Could you check a few things on this model? Use its own coordinates, in mm. A direction names the side the tool comes from. Round coordinates to 2 decimals unless told otherwise and drop trailing zeros. Loops run counter-clockwise (first coordinate to the right, second up) from the corner with the lowest first, then second, coordinate; pieces in that order, holes last. Notation, with made-up numbers: (51.25, 38) -> (92.25, 38) arc R25 ccw to (92.25, 74) -> close; hole circle Ø6 at (41.5, 17.25). An arc over 180 degrees is marked (long way). Put each result on its own line as item: value. Start each with the question number.
1. I need wall thicknesses on line 1 (Y direction, x = 134, z = 2.2); line 2 (Y direction, x = 156, z = 0.7); line 3 (Y direction, x = 65, z = 2.1). Which ranges of each line are inside material? Lowest first, please. Write a range as [from, to].
2. Imagine slicing it at C-C, the plane z = 1.3. Count the separate pieces of the cut face and the enclosed holes in it, and give its area (3 significant figures).
3. Imagine slicing it at D-D, the plane x = 124. Please give me the cut outline in (y, z) (3 decimals), and give its area (3 significant figures).
4. Imagine slicing it at A-A, the plane x = 141.5. Please give me the cut outline in (y, z) (3 decimals), and give its area (3 significant figures).
5. Which directions (+Z, -Z, +X, -X, +Y, -Y) give clear straight access to the entire face, cutting with the end or side of a thin tool? Please do faces 4 (the cylindrical face through (165.083, -51.404, 1.565)), 5 (the flat face through (148.274, 233.48, 1.61)), 6 (the cylindrical face through (84.258, 200.735, 1.565)).
6. If we mould it in two halves opening along Y, with no side actions, what happens to faces 1 (the flat face through (102, 121, 3.175)), 2 (the cylindrical face through (40.237, 288.703, 1.565)), 3 (the flat face through (56.584, 233.942, 1.61))? For each: pulls with the +Y half, pulls with the -Y half, needs draft (parallel to the pull), parting line crosses it, or undercut.
7. Imagine slicing it at B-B, the plane y = 99. Please give me the cut outline in (x, z) (3 decimals).
8. I'm going to push flat-ended pins straight in: P1, Ø1.5, axis at y = 10, z = 1, coming from the -X side; P2, Ø1.6, axis at y = 146, z = 1.5, coming from the -X side; P3, Ø1, axis at y = 134, z = 2, coming from the +X side. Where does each tip first touch, or does it pass through?
```python
from build123d import *

# Parameters (mm, degrees)
BOSS_EXTRUDE1_DEPTH = 3.175
CUT_EXTRUDE1_DEPTH  = 10
SKETCH3_R           = 2.0193
BOSS_EXTRUDE2_DEPTH = 3.175
FILLET1_R           = 10
FILLET2_R           = 50
SKETCH4_R           = 2.02
CUT_EXTRUDE2_DEPTH  = 10


with BuildPart() as part:
    # Sketch1 → Boss-Extrude1 (new body)
    with BuildSketch(Plane.XY):
        Polygon((165.934536959, -16.66935), (157.315236959, -8.05005), (115.359952094, -8.05005), (89.959952094, -8.05005), (48.004667228, -8.05005), (39.385367228, -16.66935), (39.385367228, -40.05005), (39.385367228, -52.41105), (165.934536959, -56.67505), (165.934536959, -42.05005), align=None)
        with BuildLine():
            ThreePointArc((47.685367228, -44.38075), (49.704667228, -46.40005), (47.685367228, -48.41935))
            ThreePointArc((47.685367228, -48.41935), (45.666067228, -46.40005), (47.685367228, -44.38075))
        make_face(mode=Mode.SUBTRACT)
        with BuildLine():
            ThreePointArc((47.685367228, -12.63075), (49.704667228, -14.65005), (47.685367228, -16.66935))
            ThreePointArc((47.685367228, -16.66935), (45.666067228, -14.65005), (47.685367228, -12.63075))
        make_face(mode=Mode.SUBTRACT)
        with BuildLine():
            ThreePointArc((73.085367228, -44.38075), (75.104667228, -46.40005), (73.085367228, -48.41935))
            ThreePointArc((73.085367228, -48.41935), (71.066067228, -46.40005), (73.085367228, -44.38075))
        make_face(mode=Mode.SUBTRACT)
        with BuildLine():
            ThreePointArc((73.085367228, -12.63075), (75.104667228, -14.65005), (73.085367228, -16.66935))
            ThreePointArc((73.085367228, -16.66935), (71.066067228, -14.65005), (73.085367228, -12.63075))
        make_face(mode=Mode.SUBTRACT)
        with BuildLine():
            ThreePointArc((132.234536959, -44.38075), (134.253836959, -46.40005), (132.234536959, -48.41935))
            ThreePointArc((132.234536959, -48.41935), (130.215236959, -46.40005), (132.234536959, -44.38075))
        make_face(mode=Mode.SUBTRACT)
        with BuildLine():
            ThreePointArc((132.234536959, -12.63075), (134.253836959, -14.65005), (132.234536959, -16.66935))
            ThreePointArc((132.234536959, -16.66935), (130.215236959, -14.65005), (132.234536959, -12.63075))
        make_face(mode=Mode.SUBTRACT)
        with BuildLine():
            ThreePointArc((157.634536959, -44.38075), (159.653836959, -46.40005), (157.634536959, -48.41935))
            ThreePointArc((157.634536959, -48.41935), (155.615236959, -46.40005), (157.634536959, -44.38075))
        make_face(mode=Mode.SUBTRACT)
        with BuildLine():
            ThreePointArc((157.634536959, -12.63075), (159.653836959, -14.65005), (157.634536959, -16.66935))
            ThreePointArc((157.634536959, -16.66935), (155.615236959, -14.65005), (157.634536959, -12.63075))
        make_face(mode=Mode.SUBTRACT)
        Polygon((115.359952094, -8.05005), (157.315236959, -8.05005), (115.359952094, 33.905234866), align=None)
        Polygon((89.959952094, -8.05005), (115.359952094, -8.05005), (115.359952094, 33.905234866), (115.359952094, 203.394265134), (115.359952094, 245.34955), (89.959952094, 245.34955), (89.959952094, 203.394265134), (89.959952094, 33.905234866), align=None)
        Polygon((48.004667228, -8.05005), (89.959952094, -8.05005), (89.959952094, 33.905234866), align=None)
        Polygon((89.959952094, 245.34955), (115.359952094, 245.34955), (157.315236959, 245.34955), (165.934536959, 253.96885), (165.934536959, 279.34955), (165.934536959, 293.97455), (39.385367228, 289.71055), (39.385367228, 277.34955), (39.385367228, 253.96885), (48.004667228, 245.34955), align=None)
        with BuildLine():
            ThreePointArc((47.685367228, 253.96885), (49.704667228, 251.94955), (47.685367228, 249.93025))
            ThreePointArc((47.685367228, 249.93025), (45.666067228, 251.94955), (47.685367228, 253.96885))
        make_face(mode=Mode.SUBTRACT)
        with BuildLine():
            ThreePointArc((47.685367228, 285.71885), (49.704667228, 283.69955), (47.685367228, 281.68025))
            ThreePointArc((47.685367228, 281.68025), (45.666067228, 283.69955), (47.685367228, 285.71885))
        make_face(mode=Mode.SUBTRACT)
        with BuildLine():
            ThreePointArc((73.085367228, 253.96885), (75.104667228, 251.94955), (73.085367228, 249.93025))
            ThreePointArc((73.085367228, 249.93025), (71.066067228, 251.94955), (73.085367228, 253.96885))
        make_face(mode=Mode.SUBTRACT)
        with BuildLine():
            ThreePointArc((73.085367228, 285.71885), (75.104667228, 283.69955), (73.085367228, 281.68025))
            ThreePointArc((73.085367228, 281.68025), (71.066067228, 283.69955), (73.085367228, 285.71885))
        make_face(mode=Mode.SUBTRACT)
        with BuildLine():
            ThreePointArc((132.234536959, 253.96885), (134.253836959, 251.94955), (132.234536959, 249.93025))
            ThreePointArc((132.234536959, 249.93025), (130.215236959, 251.94955), (132.234536959, 253.96885))
        make_face(mode=Mode.SUBTRACT)
        with BuildLine():
            ThreePointArc((157.634536959, 253.96885), (159.653836959, 251.94955), (157.634536959, 249.93025))
            ThreePointArc((157.634536959, 249.93025), (155.615236959, 251.94955), (157.634536959, 253.96885))
        make_face(mode=Mode.SUBTRACT)
        with BuildLine():
            ThreePointArc((157.634536959, 285.71885), (159.653836959, 283.69955), (157.634536959, 281.68025))
            ThreePointArc((157.634536959, 281.68025), (155.615236959, 283.69955), (157.634536959, 285.71885))
        make_face(mode=Mode.SUBTRACT)
        Polygon((115.359952094, 245.34955), (115.359952094, 203.394265134), (157.315236959, 245.34955), align=None)
        Polygon((48.004667228, 245.34955), (89.959952094, 203.394265134), (89.959952094, 245.34955), align=None)
    extrude(amount=BOSS_EXTRUDE1_DEPTH)

    # Sketch2 → Cut-Extrude1 (cut)
    with BuildSketch(Plane.XY.offset(3.175)):
        Polygon((84.385367228, -52.41105), (39.385367228, -52.41105), (165.934536959, -56.67505), (165.934536959, -52.41105), (120.934536959, -52.41105), align=None)
        Polygon((120.934536959, 289.71055), (165.934536959, 289.71055), (165.934536959, 293.97455), (39.385367228, 289.71055), (84.385367228, 289.71055), align=None)
    extrude(amount=-CUT_EXTRUDE1_DEPTH, mode=Mode.SUBTRACT)

    # Sketch3 → Boss-Extrude2 (add)
    with BuildSketch(Plane.XY.offset(3.175)):
        Polygon((37.385367228, -15.840922875), (37.385367228, -54.41105), (167.934536959, -54.41105), (167.934536959, -15.840922875), (117.359952094, 34.73366199), (117.359952094, 202.56583801), (167.934536959, 253.140422875), (167.934536959, 291.71055), (37.385367228, 291.71055), (37.385367228, 253.140422875), (87.959952094, 202.56583801), (87.959952094, 34.73366199), align=None)
        with Locations((132.234536959, -46.40005)):
            Circle(SKETCH3_R, mode=Mode.SUBTRACT)
        with Locations((132.234536959, -14.65005)):
            Circle(SKETCH3_R, mode=Mode.SUBTRACT)
        with Locations((47.685367228, -14.65005)):
            Circle(SKETCH3_R, mode=Mode.SUBTRACT)
        with Locations((47.685367228, -46.40005)):
            Circle(SKETCH3_R, mode=Mode.SUBTRACT)
        with Locations((73.085367228, -46.40005)):
            Circle(SKETCH3_R, mode=Mode.SUBTRACT)
        with Locations((73.085367228, -14.65005)):
            Circle(SKETCH3_R, mode=Mode.SUBTRACT)
        with Locations((157.634536959, -14.65005)):
            Circle(SKETCH3_R, mode=Mode.SUBTRACT)
        with Locations((157.634536959, -46.40005)):
            Circle(SKETCH3_R, mode=Mode.SUBTRACT)
        with Locations((132.234536959, 251.94955)):
            Circle(SKETCH3_R, mode=Mode.SUBTRACT)
        with Locations((73.085367228, 251.94955)):
            Circle(SKETCH3_R, mode=Mode.SUBTRACT)
        with Locations((157.634536959, 251.94955)):
            Circle(SKETCH3_R, mode=Mode.SUBTRACT)
        with Locations((47.685367228, 251.94955)):
            Circle(SKETCH3_R, mode=Mode.SUBTRACT)
        with Locations((47.685367228, 283.69955)):
            Circle(SKETCH3_R, mode=Mode.SUBTRACT)
        with Locations((73.085367228, 283.69955)):
            Circle(SKETCH3_R, mode=Mode.SUBTRACT)
        with Locations((157.634536959, 283.69955)):
            Circle(SKETCH3_R, mode=Mode.SUBTRACT)
    extrude(amount=-BOSS_EXTRUDE2_DEPTH)

    # Fillet1
    fillet1_edges = [part.edges().sort_by_distance(p)[0] for p in [
        (37.385367228, -54.41105, 1.5875),
        (167.934536959, -54.41105, 1.5875),
        (167.934536959, -15.840922875, 1.5875),
        (167.934536959, 253.140422875, 1.5875),
        (167.934536959, 291.71055, 1.5875),
        (37.385367228, 291.71055, 1.5875),
        (37.385367228, 253.140422875, 1.5875),
        (37.385367228, -15.840922875, 1.5875),
    ]]
    fillet(fillet1_edges, radius=FILLET1_R)

    # Fillet2
    fillet2_edges = [part.edges().sort_by_distance(p)[0] for p in [
        (117.359952094, 34.73366199, 1.5875),
        (117.359952094, 202.56583801, 1.5875),
        (87.959952094, 202.56583801, 1.5875),
        (87.959952094, 34.73366199, 1.5875),
    ]]
    fillet(fillet2_edges, radius=FILLET2_R)

    # Sketch4 → Cut-Extrude2 (cut)
    with BuildSketch(Plane.XY.offset(3.175)):
        with Locations((132.234536959, 283.69955)):
            Circle(SKETCH4_R)
    extrude(amount=-CUT_EXTRUDE2_DEPTH, mode=Mode.SUBTRACT)


solid = part.part
```
Entries:
1. line 1: [-54.41, -47.38], [-45.42, -15.63], [-13.67, 18.09], [219.21, 250.97], [252.93, 282.72], [284.68, 291.71]
1. line 2: [-54.41, -47.59], [-45.21, -15.84], [-13.46, -3.91], [241.21, 250.76], [253.14, 282.51], [284.89, 291.71]
1. line 3: [-54.41, 11.77], [225.53, 291.71]
2. separate pieces: 1
2. enclosed holes: 16
2. area: 23,000 mm^2
3. outline: (-54.411, 0) -> (30.546, 0) -> (30.546, 3.175) -> (-54.411, 3.175) -> close; (206.753, 0) -> (291.711, 0) -> (291.711, 3.175) -> (206.753, 3.175) -> close
3. area: 539 mm^2
4. outline: (-54.411, 0) -> (10.594, 0) -> (10.594, 3.175) -> (-54.411, 3.175) -> close; (226.706, 0) -> (291.711, 0) -> (291.711, 3.175) -> (226.706, 3.175) -> close
4. area: 413 mm^2
5. face 4: +Z, -Z, +X, -Y
5. face 5: +Z, -Z, +X
5. face 6: +Z, -Z, -X
6. face 1: needs draft
6. face 2: pulls with the +Y half
6. face 3: undercut
7. outline: (87.96, 0) -> (117.36, 0) -> (117.36, 3.175) -> (87.96, 3.175) -> close
8. P1: x = 62.48
8. P2: x = 87.96
8. P3: x = 117.36
